```python
from build123d import *

# Parameters (mm, degrees)
SKETCH1_R           = 9.95
BOSS_EXTRUDE1_DEPTH = 1.7
SKETCH2_R           = 1.6
CUT_EXTRUDE1_DEPTH  = 2.7
SKETCH3_W           = 11.99
SKETCH3_H           = 12
BOSS_EXTRUDE2_DEPTH = 2
SKETCH4_W           = 2
SKETCH4_H           = 2
BOSS_EXTRUDE4_DEPTH = 8
SKETCH5_W           = 5.41
SKETCH5_H           = 5.41
BOSS_EXTRUDE5_DEPTH = 1.1
SKETCH6_R           = 2
BOSS_EXTRUDE6_DEPTH = 0.1
REVOLVE1_ANGLE      = 180


with BuildPart() as part:
    # Sketch1 → Boss-Extrude1 (new body)
    with BuildSketch(Plane(origin=(0, 0, 0), x_dir=(1, 0, 0), z_dir=(0, 1, 0))):
        Circle(SKETCH1_R)
    extrude(amount=BOSS_EXTRUDE1_DEPTH)

    # Sketch2 → Cut-Extrude1 (cut, through all)
    with BuildSketch(Plane(origin=(0, 1.7, 0), x_dir=(1, 0, 0), z_dir=(0, 1, 0))):
        with Locations((9.5, 0)):
            Circle(SKETCH2_R)
        with Locations((4.75, -8.227241336)):
            Circle(SKETCH2_R)
        with Locations((-4.75, -8.227241336)):
            Circle(SKETCH2_R)
        with Locations((-9.5, 0)):
            Circle(SKETCH2_R)
        with Locations((-4.75, 8.227241336)):
            Circle(SKETCH2_R)
        with Locations((4.75, 8.227241336)):
            Circle(SKETCH2_R)
    extrude(amount=-CUT_EXTRUDE1_DEPTH, mode=Mode.SUBTRACT)

    # Sketch3 → Boss-Extrude2 (add)
    with BuildSketch(Plane(origin=(0, 1.7, 0), x_dir=(1, 0, 0), z_dir=(0, 1, 0))):
        Rectangle(SKETCH3_W, SKETCH3_H)
    extrude(amount=BOSS_EXTRUDE2_DEPTH)

    # Sketch4 → Boss-Extrude4 (add)
    with BuildSketch(Plane(origin=(0, 3.7, 0), x_dir=(1, 0, 0), z_dir=(0, 1, 0))):
        with Locations((4.995, 5)):
            Rectangle(SKETCH4_W, SKETCH4_H)
        with Locations((1.665, 5)):
            Rectangle(SKETCH4_W, SKETCH4_H)
        with Locations((-1.665, 5)):
            Rectangle(SKETCH4_W, SKETCH4_H)
        with Locations((-4.995, 5)):
            Rectangle(SKETCH4_W, SKETCH4_H)
        with Locations((1.665, 1.67)):
            Rectangle(SKETCH4_W, SKETCH4_H)
        with Locations((-1.665, 1.67)):
            Rectangle(SKETCH4_W, SKETCH4_H)
        with Locations((-4.995, 1.67)):
            Rectangle(SKETCH4_W, SKETCH4_H)
        with Locations((1.665, -1.66)):
            Rectangle(SKETCH4_W, SKETCH4_H)
        with Locations((-1.665, -1.66)):
            Rectangle(SKETCH4_W, SKETCH4_H)
        with Locations((-4.995, -1.66)):
            Rectangle(SKETCH4_W, SKETCH4_H)
        with Locations((1.665, -4.99)):
            Rectangle(SKETCH4_W, SKETCH4_H)
        with Locations((-1.665, -4.99)):
            Rectangle(SKETCH4_W, SKETCH4_H)
        with Locations((-4.995, -4.99)):
            Rectangle(SKETCH4_W, SKETCH4_H)
        with Locations((4.995, 1.67)):
            Rectangle(SKETCH4_W, SKETCH4_H)
        with Locations((4.995, -1.66)):
            Rectangle(SKETCH4_W, SKETCH4_H)
        with Locations((4.995, -4.99)):
            Rectangle(SKETCH4_W, SKETCH4_H)
    extrude(amount=BOSS_EXTRUDE4_DEPTH)

    # Sketch5 → Boss-Extrude5 (add)
    with BuildSketch(Plane(origin=(0, 0, 0), x_dir=(-1, 0, 0), z_dir=(0, -1, 0))):
        Rectangle(SKETCH5_W, SKETCH5_H)
    extrude(amount=BOSS_EXTRUDE5_DEPTH)

    # Sketch6 → Boss-Extrude6 (add)
    with BuildSketch(Plane.XZ.offset(1.1)):
        Circle(SKETCH6_R)
    extrude(amount=BOSS_EXTRUDE6_DEPTH)

    # Sketch7 → Revolve1 (revolve)
    with BuildSketch(Plane(origin=(0, -1.2, 0), x_dir=(-1, 0, 0), z_dir=(0, -1, 0))):
        with BuildLine():
            Line((0, 1.6), (0, -1.6))
            ThreePointArc((0, -1.6), (-1.6, 0), (0, 1.6))
        make_face()
    revolve(axis=Axis((0, -1.2, -1.6), (0, 0, -1)), revolution_arc=REVOLVE1_ANGLE)


solid = part.part
```
Check sheet for the modelled part. Datum: model origin and axes. Units: mm. A direction names the side the tool comes from. Give positions to 0.01 mm unless a question says otherwise; leave off trailing zeros. Order: outer loops, then holes, each group sorted by start corner. A loop starts at its lowest first (then second) coordinate and runs counter-clockwise, first axis right, second up. Notation, with made-up numbers: M 86,30 L 129,30 A34 ccw 129,64 Z; hole C 35.5,31 d9. An arc over 180 degrees is marked long. Answer in a Markdown table with one row per item. Add a question column.
Q1. Sectioned sample at D-D, the plane y = 8.25. Count the separate pieces of the cut face and the enclosed holes in it, and give its area (3 significant figures).
Q2. Sectioned sample at C-C, the plane x = 0. Record the boundary of the cut face in (y, z) (3 decimals), and give its area (3 significant figures).
Q3. Gauge pin test, flat ends, axial feed: pin 1 Ø6 at (y, z) = (7.5, -1.5) entering from +X (3 decimals); pin 2 Ø1 at (x, y) = (5.5, 8.5) entering from +Z; pin 3 Ø1 at (y, z) = (8, -8) entering from -X; pin 4 Ø2 at (x, y) = (-4.5, 8) entering from -Z. Record the tip position at first contact, or that the pin passes through.
Q4. Sectioned sample at B-B, the plane z = 0. Record the boundary of the cut face in (x, y) (3 decimals).
Q5. Release check for a two-part mould opening along Z. For faces 1 (the flat face through (5, 8, 5.99)), 2 (the flat face through (-5, 8, -0.67)), 3 (the flat face through (-2.665, 8, -2)), 4 (the flat face through (2, 8, -0.67)) record: released by +Z, released by -Z, zero draft, split by the parting line, or undercut.
Q6. Thickness scan on L1, parallel to Z at x = -1.75, y = 5; L2, parallel to X at y = 8.5, z = 5.5 (3 decimals); L3, parallel to Y at x = 3.75, z = -5.75. Record the ranges inside material, lowest first.
Q7. Sectioned sample at A-A, the plane x = -8.25. Record the boundary of the cut face in (y, z), and give its area (3 significant figures).
Q8. Access from +Z, -Z, +X, -X, +Y, -Y to the whole of each face (thin tool, end or side, straight path). Record for faces 5 (the flat face through (-5.995, 7, 1)), 6 (the flat face through (-1, 7, -6)), 7 (the flat face through (2, 8, -4)), 8 (the flat face through (5.995, 7, 1)), 9 (the flat face through (-3.995, 8, 5)).
Verdict:
| question | item | result |
|---|---|---|
| 1 | separate pieces | 16 |
| 1 | enclosed holes | 0 |
| 1 | area | 64.0 mm² |
| 2 | outline | M -1.2,-2 L -1.1,-2 L -1.1,-2.705 L 0,-2.705 L 0,-9.95 L 1.7,-9.95 L 1.7,-6 L 3.7,-6 L 3.7,6 L 1.7,6 L 1.7,9.95 L 0,9.95 L 0,2.705 L -1.1,2.705 L -1.1,2 L -1.2,2 L -1.2,1.6 A1.6 ccw -1.2,-1.6 Z |
| 2 | area | 68.2 mm² |
| 3 | pin 1 | x = 5.995 |
| 3 | pin 2 | z = 5.99 |
| 3 | pin 3 | through |
| 3 | pin 4 | z = -6 |
| 4 | outline | M -7.9,0 L -2.705,0 L -2.705,-1.1 L -2,-1.1 L -2,-1.2 L -1.6,-1.2 A1.6 ccw 1.6,-1.2 L 2,-1.2 L 2,-1.1 L 2.705,-1.1 L 2.705,0 L 7.9,0 L 7.9,1.7 L 5.995,1.7 L 5.995,3.7 L -5.995,3.7 L -5.995,1.7 L -7.9,1.7 Z |
| 5 | face 1 | released by +Z |
| 5 | face 2 | undercut |
| 5 | face 3 | zero draft |
| 5 | face 4 | undercut |
| 6 | L1 | -6 to -4, -2.67 to -0.67, 0.66 to 2.66, 3.99 to 5.99 |
| 6 | L2 | -5.995 to -3.995, -2.665 to -0.665, 0.665 to 2.665, 3.995 to 5.995 |
| 6 | L3 | 0 to 3.7 |
| 7 | outline | M 0,-5.56 L 1.7,-5.56 L 1.7,-1 L 0,-1 Z; M 0,1 L 1.7,1 L 1.7,5.56 L 0,5.56 Z |
| 7 | area | 15.5 mm² |
| 8 | face 5 | +Z, -Z, -X, +Y |
| 8 | face 6 | -Z, +X, -X, +Y |
| 8 | face 7 | +X, -X, +Y |
| 8 | face 8 | +Z, -Z, +X, +Y |
| 8 | face 9 | +Z, -Z, +Y |
